The listing builds one solid part. Answer for the finished solid, in the listing's coordinates (mm). A direction names the side the tool comes from. Coordinates: 2 decimals unless noted, no trailing zeros. Order: outer loops, then holes, each group sorted by start corner. A loop starts at its lowest first (then second) coordinate and runs counter-clockwise, first axis right, second up. Notation, with made-up numbers: (51.5, -4) -> (71.5, -4) arc R30 ccw to (71.5, 22) -> close; hole circle Ø7 at (0.5, 63.25). An arc over 180 degrees is marked (long way). Answer in a Markdown table with one row per item.
```python
from build123d import *

# Parameters (mm, degrees)
SKETCH1_R               = 2.9972
BOSS_EXTRUDE1_DEPTH     = 12.573
CUT_EXTRUDE3_DEPTH      = 62.511402554
CUT_EXTRUDE3_DEPTH_BACK = 10.9728
FILLET1_R               = 3.175
CUT_EXTRUDE1_DEPTH      = 3.429
CUT_EXTRUDE1_DEPTH_BACK = 62.511402554
SKETCH6_W               = 75.0062
SKETCH6_H               = 17.018
SKETCH6_W_2             = 41.8846
CUT_EXTRUDE4_DEPTH      = 9.398
FILLET2_R               = 0.8128


with BuildPart() as part:
    # Sketch1 → Boss-Extrude1 (new body)
    with BuildSketch(Plane(origin=(0, 0, 0), x_dir=(1, 0, 0), z_dir=(0, 1, 0))):
        with BuildLine():
            Line((-29.1688495, -45.1454495), (33.8485505, -45.1454495))
            ThreePointArc((33.8485505, -45.1454495), (38.087231389, -43.389730389), (39.8429505, -39.1510495))
            Line((39.8429505, -39.1510495), (39.8429505, 33.8485505))
            ThreePointArc((39.8429505, 33.8485505), (38.087231389, 38.087231389), (33.8485505, 39.8429505))
            Line((33.8485505, 39.8429505), (-29.1688495, 39.8429505))
            ThreePointArc((-29.1688495, 39.8429505), (-33.407530389, 38.087231389), (-35.1632495, 33.8485505))
            Line((-35.1632495, 33.8485505), (-35.1632495, -39.1510495))
            ThreePointArc((-35.1632495, -39.1510495), (-33.407530389, -43.389730389), (-29.1688495, -45.1454495))
        make_face()
        with Locations(Location((-29.1688495, 33.8485505, 0), (0, 0, 270))):
            Circle(SKETCH1_R, mode=Mode.SUBTRACT)
        with Locations(Location((33.8485505, 33.8485505, 0), (0, 0, 270))):
            Circle(SKETCH1_R, mode=Mode.SUBTRACT)
        with Locations(Location((33.8485505, -39.1510495, 0), (0, 0, 270))):
            Circle(SKETCH1_R, mode=Mode.SUBTRACT)
        with Locations(Location((-29.1688495, -39.1510495, 0), (0, 0, 270))):
            Circle(SKETCH1_R, mode=Mode.SUBTRACT)
    extrude(amount=BOSS_EXTRUDE1_DEPTH)

    # Sketch5 → Cut-Extrude3 (cut, two sides: drawn at the far end of the back side and taken through both)
    with BuildSketch(Plane(origin=(0, 12.573, 0), x_dir=(1, 0, 0), z_dir=(0, 1, 0)).offset(-CUT_EXTRUDE3_DEPTH_BACK)):
        with BuildLine():
            Line((-20.566682833, -39.1510495), (25.246383833, -39.1510495))
            ThreePointArc((25.246383833, -39.1510495), (27.061611626, -38.580962754), (28.224973399, -37.075426231))
            ThreePointArc((28.224973399, -37.075426231), (29.609869611, -34.912368611), (31.772927231, -33.527472399))
            ThreePointArc((31.772927231, -33.527472399), (33.278463754, -32.364110626), (33.8485505, -30.548882833))
            Line((33.8485505, -30.548882833), (33.8485505, 25.246383833))
            ThreePointArc((33.8485505, 25.246383833), (33.278463754, 27.061611626), (31.772927231, 28.224973399))
            ThreePointArc((31.772927231, 28.224973399), (29.637195811, 29.582718454), (28.25211412, 31.700823514))
            ThreePointArc((28.25211412, 31.700823514), (27.086350512, 33.179780767), (25.287899936, 33.738256255))
            Line((25.287899936, 33.738256255), (-20.566682833, 33.738256255))
            ThreePointArc((-20.566682833, 33.738256255), (-22.381910626, 33.168169509), (-23.545272399, 31.662632986))
            ThreePointArc((-23.545272399, 31.662632986), (-24.930168611, 29.499575366), (-27.093226231, 28.114679154))
            ThreePointArc((-27.093226231, 28.114679154), (-28.598762754, 26.951317381), (-29.1688495, 25.136089588))
            Line((-29.1688495, 25.136089588), (-29.1688495, -30.548882833))
            ThreePointArc((-29.1688495, -30.548882833), (-28.598762754, -32.364110626), (-27.093226231, -33.527472399))
            ThreePointArc((-27.093226231, -33.527472399), (-24.930168611, -34.912368611), (-23.545272399, -37.075426231))
            ThreePointArc((-23.545272399, -37.075426231), (-22.381910626, -38.580962754), (-20.566682833, -39.1510495))
        make_face()
    extrude(amount=CUT_EXTRUDE3_DEPTH + CUT_EXTRUDE3_DEPTH_BACK, mode=Mode.SUBTRACT)

    # Fillet1
    fillet1_edges = [part.edges().sort_by_distance(p)[0] for p in [
        (-22.381910626, 1.6002, -33.168169509),
        (-24.930168611, 1.6002, -29.499575366),
        (-28.598762754, 1.6002, -26.951317381),
        (-29.1688495, 1.6002, 2.706396623),
        (2.3398505, 1.6002, 39.1510495),
        (27.061611626, 1.6002, 38.580962754),
        (29.609869611, 1.6002, 34.912368611),
        (33.278463754, 1.6002, 32.364110626),
        (33.8485505, 1.6002, 2.6512495),
        (33.278463754, 1.6002, -27.061611626),
        (29.637195811, 1.6002, -29.582718454),
        (27.086350512, 1.6002, -33.179780767),
        (2.360608551, 1.6002, -33.738256255),
        (-28.598762754, 1.6002, 32.364110626),
        (-24.930168611, 1.6002, 34.912368611),
        (-22.381910626, 1.6002, 38.580962754),
    ]]
    fillet(fillet1_edges, radius=FILLET1_R)

    # Sketch2 → Cut-Extrude1 (cut, two sides: drawn at the far end of the back side and taken through both)
    with BuildSketch(Plane(origin=(0, 0, 0), x_dir=(1, 0, 0), z_dir=(0, 1, 0)).offset(-CUT_EXTRUDE1_DEPTH_BACK)):
        with BuildLine():
            Line((-4.2006495, -45.1454495), (6.2641505, -45.1454495))
            Line((6.2641505, -45.1454495), (6.2641505, 6.0609505))
            ThreePointArc((6.2641505, 6.0609505), (6.145118696, 6.348318696), (5.8577505, 6.4673505))
            Line((5.8577505, 6.4673505), (-3.7942495, 6.4673505))
            ThreePointArc((-3.7942495, 6.4673505), (-4.081617696, 6.348318696), (-4.2006495, 6.0609505))
            Line((-4.2006495, 6.0609505), (-4.2006495, -45.1454495))
        make_face()
    extrude(amount=CUT_EXTRUDE1_DEPTH + CUT_EXTRUDE1_DEPTH_BACK, mode=Mode.SUBTRACT)

    # Sketch6 → Cut-Extrude4 (cut)
    with BuildSketch(Plane(origin=(0, 12.573, 0), x_dir=(1, 0, 0), z_dir=(0, 1, 0))):
        with Locations((2.3398505, -22.1584495)):
            Rectangle(SKETCH6_W, SKETCH6_H)
        with Locations((-14.2209495, 31.3339505)):
            Rectangle(SKETCH6_W_2, SKETCH6_H)
    extrude(amount=-CUT_EXTRUDE4_DEPTH, mode=Mode.SUBTRACT)

    # Fillet2
    fillet2_edges = [part.edges().sort_by_distance(p)[0] for p in [
        (36.629380049, 3.175, 13.6494495),
        (36.628097837, 3.175, 30.6674495),
        (-31.948396837, 3.175, 30.6674495),
        (-31.949679049, 3.175, 13.6494495),
        (-31.949679049, 3.175, -22.8249505),
        (6.7213505, 3.175, -36.574232926),
    ]]
    fillet(fillet2_edges, radius=FILLET2_R)


solid = part.part
```
(1) A cutting plane is placed at D-D, the plane z = -13. Determine the outline of the cut face in (x, y) (3 decimals), then the cut area to 3 significant figures.
Check values:
| item | result |
|---|---|
| outline | (-35.163, 0) -> (39.843, 0) -> (39.843, 12.573) -> (33.849, 12.573) -> (33.849, 4.775) arc R3.175 cw to (30.674, 1.6) -> (-25.994, 1.6) arc R3.175 cw to (-29.169, 4.775) -> (-29.169, 12.573) -> (-35.163, 12.573) -> close |
| area | 256 mm² |
(2) A cutting plane is placed at B-B, the plane z = 28.5. Determine the outline of the cut face in (x, y) (3 decimals), then the cut area to 3 significant figures.
Check values:
| item | result |
|---|---|
| outline | (-35.163, 0) -> (-4.201, 0) -> (-4.201, 1.6) -> (-25.994, 1.6) arc R3.175 cw to (-28.736, 3.175) -> (-35.163, 3.175) -> close; (6.264, 0) -> (39.843, 0) -> (39.843, 3.175) -> (33.416, 3.175) arc R3.175 cw to (30.674, 1.6) -> (6.264, 1.6) -> close |
| area | 126 mm² |
(3) For a pull along X with two mould halves and no side action, classify faces 4 (the flat face through (-32, 8, 13.649)), 5 (the cylindrical face through (-28.58, 8.62, 32.39)), 6 (the flat face through (6.721, 8, -37)) as released by +X, released by -X, zero draft, split by the parting line, or undercut.
Check values:
| item | result |
|---|---|
| face 4 | zero draft |
| face 5 | undercut |
| face 6 | released by -X |
(4) A cutting plane is placed at C-C, the plane x = 8.5. Determine the outline of the cut face in (y, z) (3 decimals), then the cut area to 3 significant figures.
Check values:
| item | result |
|---|---|
| outline | (0, -39.843) -> (12.573, -39.843) -> (12.573, -33.738) -> (4.775, -33.738) arc R3.175 cw to (1.6, -30.563) -> (1.6, 35.976) arc R3.175 cw to (4.775, 39.151) -> (12.573, 39.151) -> (12.573, 45.145) -> (0, 45.145) -> close |
| area | 273 mm² |
(5) A cutting plane is placed at A-A, the plane y = 8.5. Count the separate pieces of the cut face and the enclosed holes in it, then the cut area to 3 significant figures.
Check values:
| item | result |
|---|---|
| separate pieces | 3 |
| enclosed holes | 3 |
| area | 1,240 mm² |
(6) Which of the six approach directions +Z, -Z, +X, -X, +Y, -Y give full straight-line access (tool end or side, diameter ignored) to faces 1 (the cylindrical face through (32.94, 2.55, 2.26)), 2 (the cylindrical face through (29.66, 8.62, -29.56)), 3 (the flat face through (-29.169, 9, -5))?
Check values:
| item | result |
|---|---|
| face 1 | +Y |
| face 2 | -X, +Y |
| face 3 | -Z, +Y |
(7) Find the intervals of material crossed by line 1 along X through (y, z) = (4, -14.5); line 2 along X through (y, z) = (4.75, -12.5); line 3 along Z through (x, y) = (15, 5.5), in increasing order. Write a range as from..to.
Check values:
| item | result |
|---|---|
| line 1 | -35.16..-29.07, 33.75..39.84 |
| line 2 | -35.16..-29.17, 33.85..39.84 |
| line 3 | -39.84..-33.74, 39.15..45.15 |
(8) Flat-ended cylindrical pins translate along their axes: pin 1 (0.5 mm diameter, centred on x = 1, y = 1, fed in from +Z); pin 2 (18 mm diameter, centred on x = -11.5, z = -35.5, fed in from +Y) (3 decimals); pin 3 (3 mm diameter, centred on y = 9.5, z = -36.5, fed in from -X); pin 4 (5 mm diameter, centred on x = -29.17, z = 39.15, fed in from -Y). Find the tip coordinate at first contact, or state that the pin passes through.
Check values:
| item | result |
|---|---|
| pin 1 | z = -6.47 |
| pin 2 | y = 3.175 |
| pin 3 | x = 6.72 |
| pin 4 | through |
